Geometry: final body of the model. Coordinates: model frame, mm. Face numbers are marked on the shaded views. Give positions to 0.01 mm unless a question says otherwise; leave off trailing zeros. Write each loop counter-clockwise with the first axis right and the second up, starting at its lowest first coordinate (ties: lowest second). Pieces come first, ordered by that corner, then holes. Notation, with made-up numbers: M 33,-19 L 92,-19 A17 ccw 92,5 Z; hole C 1,66.5 d2. An arc over 180 degrees is marked long. Use a Markdown table: item, result. Add a question column.
(1) Draft query along Z for the marked faces 1 and 2. Return one class per face: released by +Z, released by -Z, zero draft, split by the parting line, or undercut.
(2) Cut plane B-B (x = -16). Output: boundary loops of the cut face in (y, z).
(3) Pin query (flat end, axial travel): pin 1 Ø5 at (x, y) = (-16.5, 43.5) entering from -Z; pin 2 Ø1.5 at (y, z) = (12.5, 9) entering from -X; pin 3 Ø1 at (y, z) = (59, -31.5) entering from +X. Return the tip coordinate at first contact, or that it passes through.
(4) Cut plane C-C (z = 0). Output: boundary loops of the cut face in (x, y), plus the area to 3 significant figures.
(5) Cut plane A-A (y = 14). Output: boundary loops of the cut face in (x, z), plus the area to 3 significant figures.
(6) Cut plane D-D (x = 0). Output: boundary loops of the cut face in (y, z).
(7) Material intervals for L1, parallel to X at y = 48, z = 0; L2, parallel to Y at x = -1.5, z = -1.5; L3, parallel to Z at x = 0.5, y = 89.5, sorted ascending.
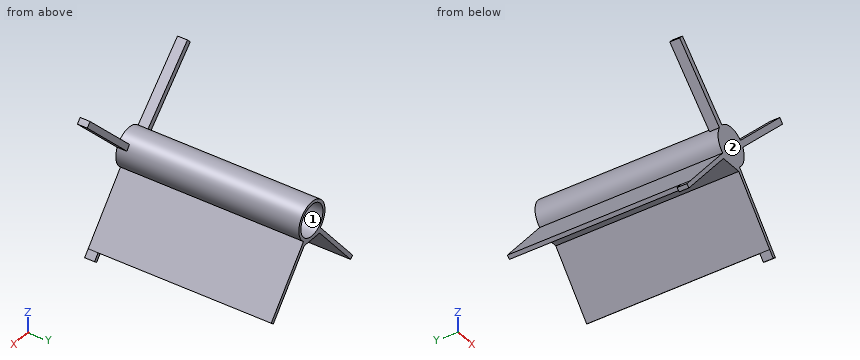
```python
from build123d import *

# Parameters (mm, degrees)
SKETCH1_R           = 9.5
BOSS_EXTRUDE1_DEPTH = 92.7
EXTRUDE_THIN1_DEPTH = 92.7
SKETCH13_W          = 2
SKETCH13_H          = 5
BOSS_EXTRUDE8_DEPTH = 5
EXTRUDE_THIN3_DEPTH = 5
SKETCH15_W          = 12.212964584
SKETCH15_H          = 2.5
BOSS_EXTRUDE9_DEPTH = 92.7
SKETCH16_R          = 8
CUT_EXTRUDE1_DEPTH  = 90
SKETCH17_R          = 55
SKETCH17_R_2        = 50
CUT_EXTRUDE2_DEPTH  = 5


with BuildPart() as part:
    # Sketch1 → Boss-Extrude1 (new body)
    with BuildSketch(Plane(origin=(0, 0, 0), x_dir=(1, 0, 0), z_dir=(0, 1, 0))):
        with Locations(Location((0, 0, 0), (0, 0, 270))):
            Circle(SKETCH1_R)
    extrude(amount=BOSS_EXTRUDE1_DEPTH)

    # Sketch2 → Extrude-Thin1 (add)
    with BuildSketch(Plane(origin=(0, 92.7, 0), x_dir=(1, 0, 0), z_dir=(0, 1, 0))):
        Polygon((0, 0), (-29.568230046, 35.238044383), (-28.036141159, 36.523619603), (1.532088886, 1.285575219), align=None)
    extrude_thin1 = extrude(amount=-EXTRUDE_THIN1_DEPTH)

    # Sketch13 → Boss-Extrude8 (add)
    with BuildSketch(Plane(origin=(-29.568230046, 0, -35.238044383), x_dir=(-0.7660444431189722, 0, 0.6427876096865464), z_dir=(-0.6427876096865464, 0, -0.7660444431189722))):
        with Locations((-1, 2.5)):
            Rectangle(SKETCH13_W, SKETCH13_H)
    boss_extrude8 = extrude(amount=BOSS_EXTRUDE8_DEPTH)

    # Mirror1: Extrude-Thin1, Boss-Extrude8 across plane
    add(extrude_thin1.mirror(Plane(origin=(0, 0, 0), x_dir=(0, 0, 1), z_dir=(1, 0, 0))))
    add(boss_extrude8.mirror(Plane(origin=(0, 0, 0), x_dir=(0, 0, 1), z_dir=(1, 0, 0))))

    # Sketch14 → Extrude-Thin3 (add)
    with BuildSketch(Plane.XZ):
        Polygon((0, 0), (36.062445841, 36.062445841), (38.183766184, 33.941125497), (2.121320344, -2.121320344), align=None)
    extrude_thin3 = extrude(amount=-EXTRUDE_THIN3_DEPTH)

    # Mirror6: Extrude-Thin3 across plane
    add(extrude_thin3.mirror(Plane(origin=(0, 0, 0), x_dir=(0, 0, 1), z_dir=(1, 0, 0))))

    # Sketch15 → Boss-Extrude9 (add)
    with BuildSketch(Plane.XZ):
        with Locations((0, -8.52742221)):
            Rectangle(SKETCH15_W, SKETCH15_H)
    extrude(amount=-BOSS_EXTRUDE9_DEPTH)

    # Sketch16 → Cut-Extrude1 (cut)
    with BuildSketch(Plane(origin=(0, 92.7, 0), x_dir=(1, 0, 0), z_dir=(0, 1, 0))):
        with Locations(Location((0, 0, 0), (0, 0, 270))):
            Circle(SKETCH16_R)
    extrude(amount=-CUT_EXTRUDE1_DEPTH, mode=Mode.SUBTRACT)

    # Sketch17 → Cut-Extrude2 (cut)
    with BuildSketch(Plane.XZ):
        Circle(SKETCH17_R)
        Circle(SKETCH17_R_2, mode=Mode.SUBTRACT)
    extrude(amount=-CUT_EXTRUDE2_DEPTH, mode=Mode.SUBTRACT)


solid = part.part
```
Answer list:
| question | item | result |
|---|---|---|
| 1 | face 1 | undercut |
| 1 | face 2 | zero draft |
| 2 | outline | M 0,-22.18 L 92.7,-22.18 L 92.7,-19.07 L 0,-19.07 Z; M 0,11.76 L 5,11.76 L 5,16 L 0,16 Z |
| 3 | pin 1 | z = -25.75 |
| 3 | pin 2 | x = -4.71 |
| 3 | pin 3 | x = 26.85 |
| 4 | outline | M -9.5,0 L 9.5,0 L 9.5,92.7 L 8,92.7 L 8,2.7 L -8,2.7 L -8,92.7 L -9.5,92.7 Z |
| 4 | area | 321 mm² |
| 5 | outline | M -29.57,-35.24 L -28.04,-36.52 L -5.59,-9.78 L 5.59,-9.78 L 28.04,-36.52 L 29.57,-35.24 L 6.11,-7.28 A9.5 ccw long -6.11,-7.28 Z; hole C 0,0 d16 |
| 5 | area | 236 mm² |
| 6 | outline | M 0,-9.78 L 92.7,-9.78 L 92.7,-8 L 2.7,-8 L 2.7,8 L 92.7,8 L 92.7,9.5 L 0,9.5 Z |
| 7 | L1 | -9.5 to -8, 8 to 9.5 |
| 7 | L2 | 0 to 2.7 |
| 7 | L3 | -9.78 to -7.98, 7.98 to 9.49 |
